from build123d import *


with BuildPart() as part:
    # Sketch1 → Revolve1 (revolve)
    with BuildSketch(Plane.XY):
        Polygon((0, 0), (29.718, 0), (29.718, 5.5499), (17.018, 5.5499), (10.668, 5.5499), (10.668, 7.62), (10.414, 7.62), (10.414, 6.858), (9.6266, 6.858), (9.6266, 7.62), (9.3726, 7.62), (9.3726, 6.858), (8.5852, 6.858), (8.5852, 7.62), (8.3312, 7.62), (8.3312, 6.858), (7.5438, 6.858), (7.5438, 7.62), (7.2898, 7.62), (7.2898, 6.858), (6.5024, 6.858), (6.5024, 7.62), (6.2484, 7.62), (6.2484, 6.858), (5.461, 6.858), (5.461, 7.62), (5.461, 8.500000018), (5.207, 8.500000018), (5.207, 7.738000018), (4.4196, 7.738000018), (4.4196, 8.500000018), (4.1656, 8.500000018), (4.1656, 7.738000018), (3.3782, 7.738000018), (3.3782, 8.500000018), (3.1242, 8.500000018), (3.1242, 7.738000018), (2.3368, 7.738000018), (2.3368, 8.500000018), (2.0828, 8.500000018), (2.0828, 7.738000018), (1.2954, 7.738000018), (1.2954, 8.500000018), (1.0414, 8.500000018), (1.0414, 7.738000018), (0.254, 7.738000018), (0.254, 8.500000018), (0, 8.500000018), align=None)
    revolve(axis=Axis((0, 0, 0), (1, 0, 0)))


solid = part.part
Could you check a few things on this model? Use its own coordinates, in mm. A direction names the side the tool comes from. Round coordinates to 2 decimals unless told otherwise and drop trailing zeros. Write each loop counter-clockwise with the first axis right and the second up, starting at its lowest first coordinate (ties: lowest second). Pieces come first, ordered by that corner, then holes. Notation, with made-up numbers: (-3.5, 69) - (15.5, 69) arc R21 cw to (15.5, 90) - close; hole circle Ø5 at (42, 79.5). An arc over 180 degrees is marked (long way). Use a Markdown table: item, result.
Q1. For faces 5 (the cylindrical face through (0.642, -1.677, -7.554)), 6 (the flat face through (29.718, 0, 0)), which set-ups out of +Z, -Z, +X, -X, +Y, -Y let a thin tool reach every point of the face, with its end or its side?
Output values:
| item | result |
|---|---|
| face 5 | none |
| face 6 | +Z, -Z, +X, +Y, -Y |
Q2. I want a section at A-A (x = 2.75). List the corners of the cut face in (y, z) for me, plus the area to 3 significant figures.
Output values:
| item | result |
|---|---|
| outline | circle Ø15.48 at (0, 0) |
| area | 188 mm2 |
Q3. Thinking about a two-plate mould opening in X: for faces 1 (the flat face through (0, 0, 0)), 2 (the flat face through (3.124, 2, -8)), 3 (the cylindrical face through (20.06, 5.127, -2.126)), 4 (the flat face through (1.295, -2, -8)), which applies, released by +X, released by -X, zero draft, split by the parting line, or undercut?
Output values:
| item | result |
|---|---|
| face 1 | released by -X |
| face 2 | undercut |
| face 3 | zero draft |
| face 4 | undercut |
Q4. Please list where these lines run through material, in increasing order: L1, parallel to X at y = 3.75, z = -7.5; L2, parallel to X at y = 6.5, z = -2.75; L3, parallel to X at y = -1.5, z = 6.5.
Output values:
| item | result |
|---|---|
| L1 | 0 to 0.25, 1.04 to 1.3, 2.08 to 2.34, 3.12 to 3.38, 4.17 to 4.42, 5.21 to 5.46 |
| L2 | 0 to 5.46, 6.25 to 6.5, 7.29 to 7.54, 8.33 to 8.59, 9.37 to 9.63, 10.41 to 10.67 |
| L3 | 0 to 10.67 |
Q5. For pin 1 (6 mm diameter, centred on x = 24.5, y = -6, fed in from +Z); pin 2 (2 mm diameter, centred on y = 5.5, z = -5, fed in from +X); pin 3 (8 mm diameter, centred on x = 20.5, z = -3, fed in from -Y), each with a flat end and sliding along its axis, tell me the tip position at first contact or that it passes through.
Output values:
| item | result |
|---|---|
| pin 1 | z = 4.67 |
| pin 2 | x = 10.67 |
| pin 3 | y = -5.55 |
